Input: dimensioned drawing with shaded views. Units: mm. Origin: part minimum x, y, z. A direction names the side the tool comes from. Give positions to 0.01 mm unless a question says otherwise; leave off trailing zeros. Write each loop counter-clockwise with the first axis right and the second up, starting at its lowest first coordinate (ties: lowest second). Pieces come first, ordered by that corner, then holes. Notation, with made-up numbers: M -23,68 L 36,68 A21 cw 36,88 Z; hole C -5.75,10.25 d6. An arc over 180 degrees is marked long. Use CSV: the item, a comma, the result in double quotes. Start each with the question number.
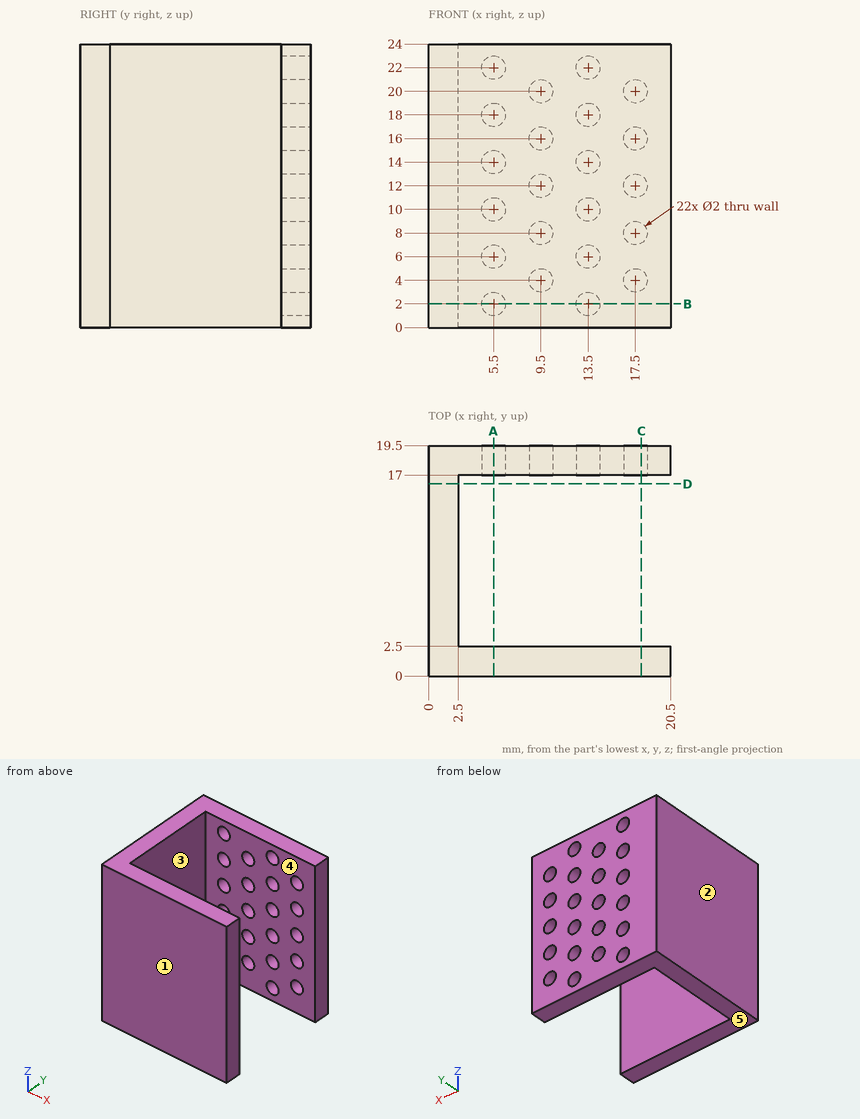
Q1. Set-up query: the marked faces 4 and 5. Return all of +Z, -Z, +X, -X, +Y, -Y with unobstructed straight access to the full face (end or side cutting, diameter ignored); none if empty.
Q2. Section D-D, the plane y = 16.25. Return the cut outline in (x, z), and give its area (3 significant figures).
Q3. Section B-B, the plane z = 2. Return the cut outline in (x, y).
Q4. Pull-direction query (Y, two-part tool) for the marked faces 1, 2 and 3; classes: released by +Y, released by -Y, zero draft, split by the parting line, or undercut.
Q5. Section A-A, the plane x = 5.5. Give the number of separate pieces and of enclosed holes in the cut face, and give its area (3 significant figures).
Q6. Material intervals for L1, parallel to X at y = 17.95, z = 14; L2, parallel to Y at x = 4.5, z = 11.75; L3, parallel to X at y = 16, z = 11, sorted ascending. Write a range as [from, to].
Q7. First-contact query: pin 1 Ø2 at (x, y) = (15, 14.5) entering from +Z. Flat tip, straight axial feed; report the tip coordinate or a pass-through.
Q8. Section C-C, the plane x = 18. Return the cut outline in (y, z), and give its area (3 significant figures).
Check result:
1,face 4,"+Z, -Z, +X"
1,face 5,"-Z, +X, -X, +Y, -Y"
2,outline,"M 0,0 L 2.5,0 L 2.5,24 L 0,24 Z"
2,area,"60.0 mm²"
3,outline,"M 0,0 L 20.5,0 L 20.5,2.5 L 2.5,2.5 L 2.5,17 L 4.5,17 L 4.5,19.5 L 0,19.5 Z; M 6.5,17 L 12.5,17 L 12.5,19.5 L 6.5,19.5 Z; M 14.5,17 L 20.5,17 L 20.5,19.5 L 14.5,19.5 Z"
4,face 1,"released by -Y"
4,face 2,"zero draft"
4,face 3,"undercut"
5,separate pieces,"8"
5,enclosed holes,"0"
5,area,"90.0 mm²"
6,L1,"x = [0, 4.5], [6.5, 12.5], [14.5, 20.5]"
6,L2,"y = [0, 2.5], [17, 19.5]"
6,L3,"x = [0, 2.5]"
7,pin 1,"passes through"
8,outline,"M 0,0 L 2.5,0 L 2.5,24 L 0,24 Z; M 17,0 L 19.5,0 L 19.5,3.13 L 17,3.13 Z; M 17,4.87 L 19.5,4.87 L 19.5,7.13 L 17,7.13 Z; M 17,8.87 L 19.5,8.87 L 19.5,11.13 L 17,11.13 Z; M 17,12.87 L 19.5,12.87 L 19.5,15.13 L 17,15.13 Z; M 17,16.87 L 19.5,16.87 L 19.5,19.13 L 17,19.13 Z; M 17,20.87 L 19.5,20.87 L 19.5,24 L 17,24 Z"
8,area,"98.3 mm²"
